Input: part model. Units: mm. Frame: model coordinates. Face numbers are marked on the shaded views. Round coordinates to 2 decimals unless told otherwise and drop trailing zeros. Loops run counter-clockwise (first coordinate to the right, second up) from the corner with the lowest first, then second, coordinate; pieces in that order, holes last. Notation, with made-up numbers: (43, -23) - (69, -23) arc R21 cw to (69, -2) - close; hole circle Ø6 at (-30.75, 22). An arc over 180 degrees is marked (long way). Write each question's results on one line, items separated by ' | '.
from build123d import *

# Parameters (mm, degrees)
BASE_DEPTH                 = 53.8
SKETCH4_R                  = 27.5
BOSS_EXTRUDE2_DEPTH        = 2
M2_CLEARANCE_HOLE1_D       = 2.6
FILLET1_R                  = 0.5
SIDE_HOLES_D               = 3.2
SIDE_ARM_DEPTH             = 10
F_3_2_3_2_DIAMETER_HOLE1_D = 3.2
FILLET2_R                  = 1


with BuildPart() as part:
    # Sketch1 → Base (new, symmetric)
    with BuildSketch(Plane.XY):
        Polygon((8, 4), (-8, 4), (0, -4), (8, -4), align=None)
    extrude(amount=BASE_DEPTH, both=True)

    # Sketch4 → Boss-Extrude2 (add)
    with BuildSketch(Plane(origin=(-2, -2, 0), x_dir=(0, 0, 1), z_dir=(-0.7071067811865475, -0.7071067811865476, 0))):
        with Locations((0, 2.828427125)):
            Circle(SKETCH4_R)
    extrude(amount=-BOSS_EXTRUDE2_DEPTH)

    # M2 Clearance Hole1 (through all)
    with Locations(Plane(origin=(-0.585786438, -0.585786438, 0), x_dir=(0.7071067811865475, -0.7071067811865477, 0), z_dir=(0.7071067811865477, 0.7071067811865475, 0))):
        with Locations((-23.828427125, 0), (11.171572875, 21), (11.171572875, -21)):
            Hole(M2_CLEARANCE_HOLE1_D / 2)

    # Sketch8 → Revolve1 (revolve)
    with BuildSketch(Plane(origin=(-2, 2, 0), x_dir=(0, 0, 1), z_dir=(0.7071067811865437, -0.7071067811865515, 0))):
        with BuildLine():
            Line((0, 3.828427125), (0, 2.828427125))
            Line((0, 2.828427125), (-12, 2.828427125))
            Line((-12, 2.828427125), (-6.5, 10.328427125))
            ThreePointArc((-6.5, 10.328427125), (-4.596194078, 5.732233047), (0, 3.828427125))
        make_face()
    revolve(axis=Axis((-4, 0, 0), (-0.7071067811865515, -0.7071067811865437, 0)))

    # Fillet1
    fillet1_edges = [part.edges().sort_by_distance(p)[0] for p in [
        (-9.303300859, -5.303300859, 6.5),
    ]]
    fillet(fillet1_edges, radius=FILLET1_R)

    # Side Holes (through all)
    with Locations(Plane.XY.offset(53.8)):
        with Locations((0, 0.5)):
            Hole(SIDE_HOLES_D / 2)

    # Sketch9 → Side Arm (add)
    with BuildSketch(Plane.XY.offset(53.8)):
        Polygon((-8, 4), (0, -4), (-37, -4), (-37, 4), align=None)
    side_arm = extrude(amount=-SIDE_ARM_DEPTH)

    # Mirror1: Side Arm across plane
    add(side_arm.mirror(Plane.XY))

    # Ø3.2 (3.2) Diameter Hole1 (through all)
    with Locations(Plane.XY.offset(53.8)):
        with Locations((-30, 0.5)):
            Hole(F_3_2_3_2_DIAMETER_HOLE1_D / 2)

    # Fillet2
    fillet2_edges = [part.edges().sort_by_distance(p)[0] for p in [
        (8, 4, 0),
    ]]
    fillet(fillet2_edges, radius=FILLET2_R)


solid = part.part
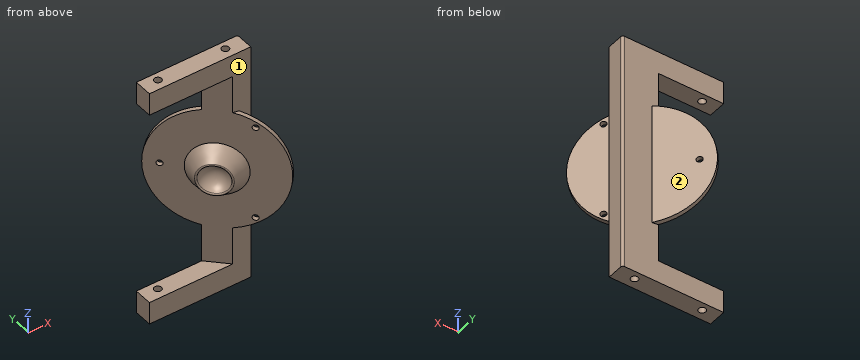
1. Contact query for flat-ended pins moving along their axis: pin 1 (6 mm diameter, centred on x = 4, z = -19, fed in from +Y); pin 2 (1 mm diameter, centred on y = 14, z = -3, fed in from -X); pin 3 (4 mm diameter, centred on y = 11.5, z = -4.5, fed in from -X). Output: stop coordinate, or through.
Answer:
pin 1: y = 4 | pin 2: x = -18.5 | pin 3: x = -17.5
2. Line query: line 1 (Y direction, x = 0, z = 14); line 2 (Z direction, x = -26.5, y = 0.5); line 3 (X direction, y = -3, z = 1.5). Output: solid intervals per line, ascending. Write a range as [from, to].
Answer:
line 1: [-4, -1.1], [2.1, 4] | line 2: [-53.8, -43.8], [43.8, 53.8] | line 3: [-3.41, 8]
3. Section query A-A, the plane x = -30. Output: boundary loops of the cut face in (y, z), plus the area to 3 significant figures.
Answer:
outline: (-4, -53.8) - (-1.1, -53.8) - (-1.1, -43.8) - (-4, -43.8) - close; (-4, 43.8) - (-1.1, 43.8) - (-1.1, 53.8) - (-4, 53.8) - close; (2.1, -53.8) - (4, -53.8) - (4, -43.8) - (2.1, -43.8) - close; (2.1, 43.8) - (4, 43.8) - (4, 53.8) - (2.1, 53.8) - close | area: 96.0 mm^2
4. Section query B-B, the plane z = 38.5. Output: boundary loops of the cut face in (x, y).
Answer:
outline: (-8, 4) - (0, -4) - (8, -4) - (8, 3) arc R1 ccw to (7, 4) - close; hole circle Ø3.2 at (0, 0.5)
5. Mould query, pull axis Y, two halves, no side actions, for the marked faces 1 and 2. Classes: pulls with the +Y half, pulls with the -Y half, needs draft (parallel to the pull), parting line crosses it, or undercut.
Answer:
face 1: undercut | face 2: pulls with the +Y half
